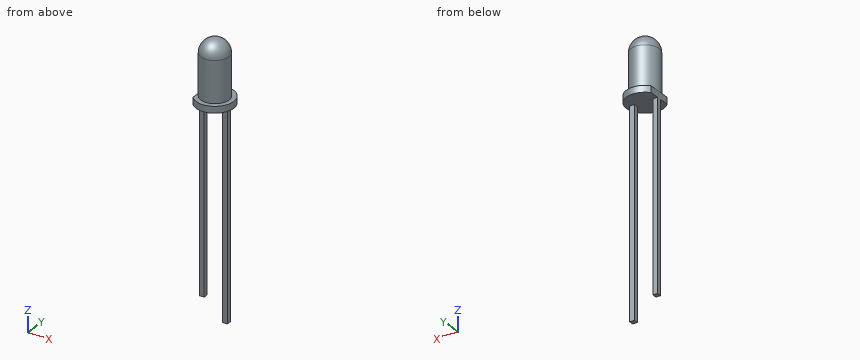
from build123d import *

# Parameters (mm, degrees)
F0_R      = 1.5
F1_DEPTH  = 5.1
F5_DEPTH  = 0.7
F6_W      = 0.5
F6_H      = 0.5
F7_DEPTH  = 20
F7_FACE_W = 0.5
F7_FACE_H = 0.5
F8_DEPTH  = 2


with BuildPart() as f1:
    # F0 (on Top) → F1 (new body)
    with BuildSketch(Plane.XY):
        Circle(F0_R)
    extrude(amount=F1_DEPTH)

    # F2 (on face) → F3 (revolve)
    with BuildSketch(Plane.XY.offset(5.1)):
        with BuildLine():
            ThreePointArc((0, 1.5), (-1.5, 0), (0, -1.5))
            Line((0, -1.5), (0, 1.5))
        make_face()
    revolve(axis=Axis((0, 0, 5.1), (0, 1, 0)))

    # F4 (on face) → F5 (join)
    with BuildSketch(Plane(origin=(0, 0, 0), x_dir=(1, 0, 0), z_dir=(0, 0, -1))):
        with BuildLine():
            Line((-1.5, 1.322876), (-1.5, -1.322876))
            ThreePointArc((-1.5, -1.322876), (2, 0), (-1.5, 1.322876))
        make_face()
    extrude(amount=-F5_DEPTH)

    # F6 (on face) → F7 (join)
    with BuildSketch(Plane(origin=(0, 0, 0), x_dir=(1, 0, 0), z_dir=(0, 0, -1))):
        with Locations((1.25, 0)):
            Rectangle(F6_W, F6_H)
        with Locations((-1.25, 0)):
            Rectangle(F6_W, F6_H)
    extrude(amount=F7_DEPTH)

    # F7_face (on face) → F8 (join)
    with BuildSketch(Plane(origin=(1.25, 0, -20), x_dir=(1, 0, 0), z_dir=(0, 0, -1))):
        Rectangle(F7_FACE_W, F7_FACE_H)
    extrude(amount=F8_DEPTH)


solid = f1.part
CAD build for the part. Positions are in the model's coordinates, mm. Coordinates: 2 decimals unless noted, no trailing zeros. Write each loop counter-clockwise with the first axis right and the second up, starting at its lowest first coordinate (ties: lowest second). Pieces come first, ordered by that corner, then holes. Notation, with made-up numbers: M 29.5,1.5 L 47.5,1.5 A26 ccw 47.5,24.5 Z; hole C 0,39.5 d9. An arc over 180 degrees is marked long. Answer as a JSON object with one key per item and string values. Group by question number.
1) Saw through at D-D (z = 4.25). Write the cut outline in (x, y), plus the area to 3 significant figures.
2) Saw through at B-B (x = 0). Write the cut outline in (y, z).
3) Pin check, flat tips, straight feed: pin 1 Ø1 at (y, z) = (0.5, -5) entering from +X; pin 2 Ø0.6 at (x, z) = (-1, -10) entering from +Y. Stop position of each tip, or through.
4) Wall check: line 1 (X direction, y = 0, z = -6); line 2 (Y direction, x = 1.1, z = -12); line 3 (Z direction, x = -1.2, y = -1.4). Give the ranges that are in metal, low to high. Write a range as from..to.
5) Saw through at A-A (z = -5.25). Write the cut outline in (x, y).
6) Saw through at C-C (y = -0.7). Write the cut outline in (x, z).
Values follow:
{
 "1": {"outline": "C 0,0 d3", "area": "7.07 mm2"},
 "2": {"outline": "M -2,0 L 2,0 L 2,0.7 L 1.5,0.7 L 1.5,5.1 A1.5 ccw -1.5,5.1 L -1.5,0.7 L -2,0.7 Z"},
 "3": {"pin 1": "stops at x = 1.5", "pin 2": "stops at y = 0.25"},
 "4": {"line 1": "x = -1.5..-1, 1..1.5", "line 2": "y = -0.25..0.25", "line 3": "z = 0..0.7"},
 "5": {"outline": "M -1.5,-0.25 L -1,-0.25 L -1,0.25 L -1.5,0.25 Z; M 1,-0.25 L 1.5,-0.25 L 1.5,0.25 L 1,0.25 Z"},
 "6": {"outline": "M -1.5,0 L 1.87,0 L 1.87,0.7 L 1.33,0.7 L 1.33,5.1 A1.33 ccw -1.33,5.1 L -1.33,0.7 L -1.5,0.7 Z"}
}
